```python
from build123d import *

# Parameters (mm, degrees)
SKETCH1_W           = 24
SKETCH1_H           = 24
BOSS_EXTRUDE1_DEPTH = 4
SKETCH2_W           = 3
SKETCH2_H           = 24
BOSS_EXTRUDE2_DEPTH = 28
SKETCH3_R           = 2.75
SKETCH3_R_2         = 0.9
CUT_EXTRUDE1_DEPTH  = 3
SKETCH4_R           = 1.7
CUT_EXTRUDE2_DEPTH  = 4
SKETCH6_W           = 12
SKETCH6_H           = 2
BOSS_EXTRUDE3_DEPTH = 11


with BuildPart() as part:
    # Sketch1 → Boss-Extrude1 (new body)
    with BuildSketch(Plane(origin=(0, 0, 0), x_dir=(1, 0, 0), z_dir=(0, 1, 0))):
        Rectangle(SKETCH1_W, SKETCH1_H)
    extrude(amount=BOSS_EXTRUDE1_DEPTH)

    # Sketch2 → Boss-Extrude2 (add)
    with BuildSketch(Plane(origin=(0, 4, 0), x_dir=(1, 0, 0), z_dir=(0, 1, 0))):
        with Locations((-10.5, 0)):
            Rectangle(SKETCH2_W, SKETCH2_H)
    extrude(amount=BOSS_EXTRUDE2_DEPTH)

    # Sketch3 → Cut-Extrude1 (cut)
    with BuildSketch(Plane(origin=(-9, 0, 0), x_dir=(0, 0, -1), z_dir=(1, 0, 0))):
        with Locations((0, 22)):
            Circle(SKETCH3_R)
        with Locations((4.5, 22)):
            Circle(SKETCH3_R_2)
        with Locations((-4.5, 22)):
            Circle(SKETCH3_R_2)
    extrude(amount=-CUT_EXTRUDE1_DEPTH, mode=Mode.SUBTRACT)

    # Sketch4 → Cut-Extrude2 (cut)
    with BuildSketch(Plane(origin=(0, 4, 0), x_dir=(1, 0, 0), z_dir=(0, 1, 0))):
        with Locations(Location((2, 6, 0), (0, 0, 270))):
            Circle(SKETCH4_R)
        with Locations(Location((2, -6, 0), (0, 0, 270))):
            Circle(SKETCH4_R)
    extrude(amount=-CUT_EXTRUDE2_DEPTH, mode=Mode.SUBTRACT)

    # Sketch6 → Boss-Extrude3 (add)
    with BuildSketch(Plane(origin=(0, 4, 0), x_dir=(1, 0, 0), z_dir=(0, 1, 0))):
        with Locations((-3, -10)):
            Rectangle(SKETCH6_W, SKETCH6_H)
        with Locations((-3, 10)):
            Rectangle(SKETCH6_W, SKETCH6_H)
    extrude(amount=BOSS_EXTRUDE3_DEPTH)


solid = part.part
```
For this review, take the finished solid that the model builds, in its own axes (mm). A direction names the side the tool comes from. Give positions to 0.01 mm unless a question says otherwise; leave off trailing zeros. Write each loop counter-clockwise with the first axis right and the second up, starting at its lowest first coordinate (ties: lowest second). Pieces come first, ordered by that corner, then holes. Notation, with made-up numbers: M 30.5,26 L 61.5,26 A17 cw 61.5,58 Z; hole C 58.25,-30.5 d11. An arc over 180 degrees is marked long. One line per item, written item: value.
1) Take a section at A-A, the plane y = 22. Write out the cut boundary in (x, z), then the cut area to 3 significant figures.
Results are:
outline: M -12,-12 L -9,-12 L -9,-5.4 L -12,-5.4 Z; M -12,-3.6 L -9,-3.6 L -9,-2.75 L -12,-2.75 Z; M -12,2.75 L -9,2.75 L -9,3.6 L -12,3.6 Z; M -12,5.4 L -9,5.4 L -9,12 L -12,12 Z
area: 44.7 mm²
2) For line 1 (Y direction, x = -10.35, z = -4.5); line 2 (Z direction, x = 0.5, y = 10); line 3 (X direction, y = 21, z = 10.25), list the stretches that pass through material, from the lowest coordinate up. Write a range as from..to.
Results are:
line 1: y = 0..21.1, 22.9..32
line 2: z = -11..-9, 9..11
line 3: x = -12..-9
3) The part is to be moulded in two halves that separate along Y. For faces 4 (the cylindrical face through (-10.48, 22.89, -4.38)), 5 (the flat face through (-3, 9, -9)), 6 (the flat face through (-3, 15, 10)), say which applies: +Y half, -Y half, draft (parallel to the pull), parting line (faces both ways), or undercut.
Results are:
face 4: undercut
face 5: draft
face 6: +Y half
4) Take a section at B-B, the plane z = 0. Write out the cut boundary in (x, y), then the cut area to 4 significant figures.
Results are:
outline: M -12,0 L 12,0 L 12,4 L -9,4 L -9,19.25 L -12,19.25 Z; M -12,24.75 L -9,24.75 L -9,32 L -12,32 Z
area: 163.5 mm²
5) Take a section at D-D, the plane x = -7.25. Write out the cut boundary in (y, z).
Results are:
outline: M 0,-12 L 4,-12 L 4,-11 L 15,-11 L 15,-9 L 4,-9 L 4,9 L 15,9 L 15,11 L 4,11 L 4,12 L 0,12 Z
6) For P1, Ø5, axis at y = 27.5, z = 1, coming from the +X side; P2, Ø3, axis at x = -1, z = -9, coming from the +Y side; P3, Ø5.5, axis at x = -6, y = 10, coming from the -Z side, all flat-tipped, find the tip position at first contact; note any pin that passes through.
Results are:
P1: stops at x = -9
P2: stops at y = 15
P3: stops at z = -11
7) For faces 1 (the flat face through (-3, 9, 9)), 2 (the flat face through (-3, 9, 11)), 3 (the flat face through (3, 9, 10)), list the 3-axis set-ups (+Z, -Z, +X, -X, +Y, -Y) from which the entire face can be reached by the end or side of a thin tool; tool diameter is ignored.
Results are:
face 1: +X, +Y
face 2: +Z, +X, +Y
face 3: +Z, -Z, +X, +Y
8) Take a section at C-C, the plane x = 2. Write out the cut boundary in (y, z).
Results are:
outline: M 0,-12 L 4,-12 L 4,-11 L 15,-11 L 15,-9 L 4,-9 L 4,-7.7 L 0,-7.7 Z; M 0,-4.3 L 4,-4.3 L 4,4.3 L 0,4.3 Z; M 0,7.7 L 4,7.7 L 4,9 L 15,9 L 15,11 L 4,11 L 4,12 L 0,12 Z
